The model under review builds one solid part; all positions refer to its coordinate system, in mm. Give positions to 0.01 mm unless a question says otherwise; leave off trailing zeros. Order: outer loops, then holes, each group sorted by start corner. A loop starts at its lowest first (then second) coordinate and runs counter-clockwise, first axis right, second up. Notation, with made-up numbers: (41.25, -21) - (94.25, -21) arc R30 ccw to (94.25, 4) - close; hole circle Ø1 at (-4.5, -34.75). An arc over 180 degrees is marked (long way). Use a Markdown table: item, result. Add a question column.
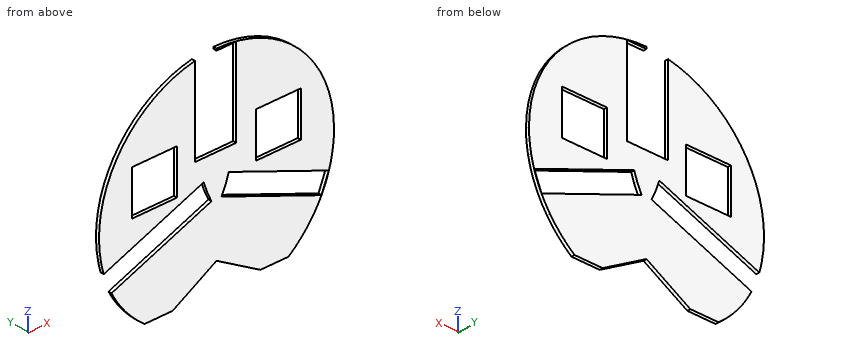
```python
from build123d import *

# Parameters (mm, degrees)
F0_W     = 40
F0_H     = 40
F1_DEPTH = 3


with BuildPart() as f1:
    # F0 (on Front) → F1 (new body)
    with BuildSketch(Plane.XZ):
        with BuildLine():
            ThreePointArc((103.0776406404, -20), (104.5183052562, -10.0460871177), (105, 0))
            ThreePointArc((105, 0), (74.2462120246, 74.2462120246), (0, 105))
            Line((0, 105), (0, 103.22223589))
            Line((0, 103.22223589), (17.5601970418, 103.22223589))
            Line((17.5601970418, 103.22223589), (17.5601970418, 24.52223589))
            Line((17.5601970418, 24.52223589), (0, 24.52223589))
            Line((0, 24.52223589), (0, 0))
            Line((0, 0), (0, -20))
            Line((0, -20), (24.9232704506, -20))
            Line((24.9232704506, -20), (4.4912775015, -11.950507217))
            Line((4.4912775015, -11.950507217), (8.3736020394, -3.2989072261))
            Line((8.3736020394, -3.2989072261), (10.9988783344, 4.5677080197))
            Line((10.9988783344, 4.5677080197), (73.3589860543, -20))
            Line((73.3589860543, -20), (103.0776406404, -20))
        make_face()
        with Locations((55.2959036827, 23.426694544)):
            Rectangle(F0_W, F0_H, mode=Mode.SUBTRACT)
        with BuildLine():
            Line((-19.2398029582, 24.52223589), (-19.2398029582, 103.22223589))
            ThreePointArc((-19.2398029582, 103.22223589), (-86.8119755941, 59.06505645), (-103.0776406404, -20))
            Line((-103.0776406404, -20), (-76.6085577032, -20))
            Line((-76.6085577032, -20), (-11.4596459847, 5.666399553))
            Line((-11.4596459847, 5.666399553), (-8.3736020394, -3.2989072261))
            Line((-8.3736020394, -3.2989072261), (-4.5281557545, -11.9277723195))
            Line((-4.5281557545, -11.9277723195), (-25.0178565965, -20))
            Line((-25.0178565965, -20), (0, -20))
            Line((0, -20), (0, 0))
            Line((0, 0), (0, 24.52223589))
            Line((0, 24.52223589), (-19.2398029582, 24.52223589))
        make_face()
        with Locations((-55.2958999333, 23.426694544)):
            Rectangle(F0_W, F0_H, mode=Mode.SUBTRACT)
        with BuildLine():
            Line((-76.6085577032, -20), (-103.0776406404, -20))
            ThreePointArc((-103.0776406404, -20), (-102.0327301186, -24.7855196543), (-100.7657719775, -29.5171000911))
            Line((-100.7657719775, -29.5171000911), (-76.6085577032, -20))
        make_face()
        with BuildLine():
            ThreePointArc((86.1684396981, -60), (96.7135964116, -40.8837408896), (103.0776406404, -20))
            Line((103.0776406404, -20), (73.3589860543, -20))
            Line((73.3589860543, -20), (100.3173000877, -30.6206357252))
            Line((100.3173000877, -30.6206357252), (97.2817984504, -38.3256364902))
            Line((97.2817984504, -38.3256364902), (93.8096992547, -47.138850962))
            Line((93.8096992547, -47.138850962), (24.9232704506, -20))
            Line((24.9232704506, -20), (0, -20))
            Line((0, -20), (86.1684396981, -60))
        make_face()
        with BuildLine():
            Line((-86.1684396981, -60), (0, -20))
            Line((0, -20), (-25.0178565965, -20))
            Line((-25.0178565965, -20), (-93.837198319, -47.1124209911))
            ThreePointArc((-93.837198319, -47.1124209911), (-90.2331970655, -53.6932970429), (-86.1684396981, -60))
        make_face()
        with BuildLine():
            ThreePointArc((64.3189255464, -82.9944324432), (76.1170004362, -72.3270505731), (86.1684396981, -60))
            Line((86.1684396981, -60), (0, -20))
            Line((0, -20), (-86.1684396981, -60))
            ThreePointArc((-86.1684396981, -60), (-76.1170004362, -72.3270505731), (-64.3189255464, -82.9944324432))
            Line((-64.3189255464, -82.9944324432), (-39.1973913604, -82.9944324432))
            Line((-39.1973913604, -82.9944324432), (0, -60))
            Line((0, -60), (39.1975319574, -82.9944324432))
            Line((39.1975319574, -82.9944324432), (64.3189255464, -82.9944324432))
        make_face()
    extrude(amount=F1_DEPTH)


solid = f1.part
```
Q1. We need section D-D (z = 15.5). Write out the cut boundary in (x, y).
Q2. We need section A-A (z = 35). Write out the cut boundary in (x, y), plus the area to 3 significant figures.
Q3. We need section B-B (x = 31). Write out the cut boundary in (y, z), plus the area to 3 significant figures.
Q4. Wall thickness on probe 1 along Z at (x, y) = (47, -1.9); probe 2 along Z at (x, y) = (43.5, -2.2); probe 3 along X at (y, z) = (-0.95, 39): over which ranges is each line inside the solid? List them lowest first.
Q5. We need section C-C (z = 85). Write out the cut boundary in (x, y).
Q6. Clearance check with flat-ended pins moving along their axes: P1, Ø1.5, axis at x = -52, y = -1, coming from the +Z side; P2, Ø0.9, axis at y = -1, z = 63, coming from the -X side; P3, Ø1.5, axis at y = -1.5, z = 23, coming from the +X side. State where each tip first meets the part, or that it passes through.
Here are the results:
| question | item | result |
|---|---|---|
| 1 | outline | (-103.85, -3) - (-75.3, -3) - (-75.3, 0) - (-103.85, 0) - close; (-35.3, -3) - (35.3, -3) - (35.3, 0) - (-35.3, 0) - close; (75.3, -3) - (103.85, -3) - (103.85, 0) - (75.3, 0) - close |
| 2 | outline | (-98.99, -3) - (-75.3, -3) - (-75.3, 0) - (-98.99, 0) - close; (-35.3, -3) - (-19.24, -3) - (-19.24, 0) - (-35.3, 0) - close; (17.56, -3) - (35.3, -3) - (35.3, 0) - (17.56, 0) - close; (75.3, -3) - (98.99, -3) - (98.99, 0) - (75.3, 0) - close |
| 2 | area | 244 mm2 |
| 3 | outline | (-3, -78.19) - (0, -78.19) - (0, -22.39) - (-3, -22.39) - close; (-3, -3.31) - (0, -3.31) - (0, 100.32) - (-3, 100.32) - close |
| 3 | area | 478 mm2 |
| 4 | probe 1 | -82.99 to -28.7, -9.62 to 3.43, 43.43 to 93.89 |
| 4 | probe 2 | -82.99 to -27.32, -8.24 to 3.43, 43.43 to 95.57 |
| 4 | probe 3 | -97.49 to -75.3, -35.3 to -19.24, 17.56 to 35.3, 75.3 to 97.49 |
| 5 | outline | (-61.64, -3) - (-19.24, -3) - (-19.24, 0) - (-61.64, 0) - close; (17.56, -3) - (61.64, -3) - (61.64, 0) - (17.56, 0) - close |
| 6 | P1 | z = 91.64 |
| 6 | P2 | x = -84.34 |
| 6 | P3 | x = 102.62 |
